```python
from build123d import *

# Parameters (mm, degrees)
SKETCH_1_W          = 35
SKETCH_1_H          = 43.5
EXTRUDE_1_DEPTH     = 20
SKETCH_2_W          = 20
SKETCH_2_H          = 5
EXTRUDE_2_DEPTH     = 10
SKETCH_3_W          = 20
SKETCH_3_H          = 5
EXTRUDE_3_DEPTH     = 10
SKETCH_4_R          = 1.5
CUT_EXTRUDE_2_DEPTH = 5
SKETCH_5_R          = 12.7
CUT_EXTRUDE_3_DEPTH = 20


with BuildPart() as part:
    # Эскиз1 → Бобышка-Вытянуть1 (new body)
    with BuildSketch(Plane.XY):
        Rectangle(SKETCH_1_W, SKETCH_1_H)
    extrude(amount=EXTRUDE_1_DEPTH)

    # Эскиз2 → Бобышка-Вытянуть2 (add)
    with BuildSketch(Plane(origin=(17.5, 0, 0), x_dir=(0, 0, -1), z_dir=(1, 0, 0))):
        with Locations((-10, -19.25)):
            Rectangle(SKETCH_2_W, SKETCH_2_H)
    extrude(amount=EXTRUDE_2_DEPTH)

    # Эскиз3 → Бобышка-Вытянуть3 (add)
    with BuildSketch(Plane.ZY.offset(17.5)):
        with Locations((10, -19.25)):
            Rectangle(SKETCH_3_W, SKETCH_3_H)
    extrude(amount=EXTRUDE_3_DEPTH)

    # Эскиз4 → Вырез-Вытянуть2 (cut)
    with BuildSketch(Plane(origin=(0, -16.75, 0), x_dir=(1, 0, 0), z_dir=(0, 1, 0))):
        with Locations((-22.5, -16)):
            Circle(SKETCH_4_R)
        with Locations((-22.5, -4)):
            Circle(SKETCH_4_R)
        with Locations((22.5, -16)):
            Circle(SKETCH_4_R)
        with Locations((22.5, -4)):
            Circle(SKETCH_4_R)
    extrude(amount=-CUT_EXTRUDE_2_DEPTH, mode=Mode.SUBTRACT)

    # Эскиз5 → Вырез-Вытянуть3 (cut)
    with BuildSketch(Plane(origin=(0, 0, 0), x_dir=(-1, 0, 0), z_dir=(0, 0, -1))):
        with Locations((0, 8.25)):
            Circle(SKETCH_5_R)
    extrude(amount=-CUT_EXTRUDE_3_DEPTH, mode=Mode.SUBTRACT)


solid = part.part
```
The listing builds one solid part. Answer for the finished solid, in the listing's coordinates (mm). A direction names the side the tool comes from. Round coordinates to 2 decimals unless told otherwise and drop trailing zeros. Write each loop counter-clockwise with the first axis right and the second up, starting at its lowest first coordinate (ties: lowest second). Pieces come first, ordered by that corner, then holes. Notation, with made-up numbers: (35.25, -36.5) -> (66.25, -36.5) arc R21 cw to (66.25, 1.5) -> close; hole circle Ø6 at (42.5, -30.75). An arc over 180 degrees is marked (long way). Use CSV: the item, a comma, the result in double quotes. Start each with the question number.
(1) Section C-C on z = 11.25 is taken. Give the vertices of the cut face in (x, y), then the cut area to 3 significant figures.
(2) Consider L1, parallel to Z at x = -22.5, y = -17.75; L2, parallel to X at y = -19.9, z = 16; L3, parallel to Z at x = 22, y = -17. Determine where each line is inside the solid, lowest interval first. Write a range as from..to.
(3) Which of the six approach directions +Z, -Z, +X, -X, +Y, -Y give full straight-line access (tool end or side, diameter ignored) to faces 5 (the face through (22, -16.75, 10)), 6 (the face through (0, -10, 20))?
(4) Each of these flat-tipped pins is pushed along its axis until it touches: pin 1 (6 mm diameter, centred on y = -1, z = 7, fed in from -X); pin 2 (10 mm diameter, centred on y = 1, z = 10, fed in from +X); pin 3 (5 mm diameter, centred on x = 22.5, z = 16, fed in from +Y). Where does it stop, or does it pass through?
(5) The mould has two halves that part along X. Classify faces 1 (the face through (-17.5, 2, 10)), 2 (the face through (-24, -19, 16)), 3 (the face through (-22, -16.75, 10)), 4 (the face through (27.5, -19, 10)): released by +X, released by -X, zero draft, split by the parting line, or undercut.
(6) Section A-A on z = 16 is taken. Give the vertices of the cut face in (x, y), then the cut area to 3 significant figures.
(7) Section B-B on x = -22.5 is taken. Give the vertices of the cut face in (y, z).
(8) Section D-D on y = 17 is taken. Give the vertices of the cut face in (x, z), then the cut area to 3 significant figures.
A:
1,outline,"(-27.5, -21.75) -> (27.5, -21.75) -> (27.5, -16.75) -> (17.5, -16.75) -> (17.5, 21.75) -> (-17.5, 21.75) -> (-17.5, -16.75) -> (-27.5, -16.75) -> close; hole circle Ø25.4 at (0, 8.25)"
1,area,"1,120 mm²"
2,L1,"z = 0..2.5, 5.5..14.5, 17.5..20"
2,L2,"x = -27.5..-24, -21..21, 24..27.5"
2,L3,"z = 0..2.59, 5.41..14.59, 17.41..20"
3,face 5,"+Z, -Z, +X, +Y"
3,face 6,"+Z, +X, -X, +Y, -Y"
4,pin 1,"stops at x = -17.5"
4,pin 2,"stops at x = 17.5"
4,pin 3,"stops at y = -16.75"
5,face 1,"released by -X"
5,face 2,"undercut"
5,face 3,"zero draft"
5,face 4,"released by +X"
6,outline,"(-27.5, -21.75) -> (-24, -21.75) -> (-24, -16.75) -> (-27.5, -16.75) -> close; (-21, -21.75) -> (21, -21.75) -> (21, -16.75) -> (17.5, -16.75) -> (17.5, 21.75) -> (-17.5, 21.75) -> (-17.5, -16.75) -> (-21, -16.75) -> close; (24, -21.75) -> (27.5, -21.75) -> (27.5, -16.75) -> (24, -16.75) -> close; hole circle Ø25.4 at (0, 8.25)"
6,area,"1,090 mm²"
7,outline,"(-21.75, 0) -> (-16.75, 0) -> (-16.75, 2.5) -> (-21.75, 2.5) -> close; (-21.75, 5.5) -> (-16.75, 5.5) -> (-16.75, 14.5) -> (-21.75, 14.5) -> close; (-21.75, 17.5) -> (-16.75, 17.5) -> (-16.75, 20) -> (-21.75, 20) -> close"
8,outline,"(-17.5, 0) -> (-9.2, 0) -> (-9.2, 20) -> (-17.5, 20) -> close; (9.2, 0) -> (17.5, 0) -> (17.5, 20) -> (9.2, 20) -> close"
8,area,"332 mm²"
